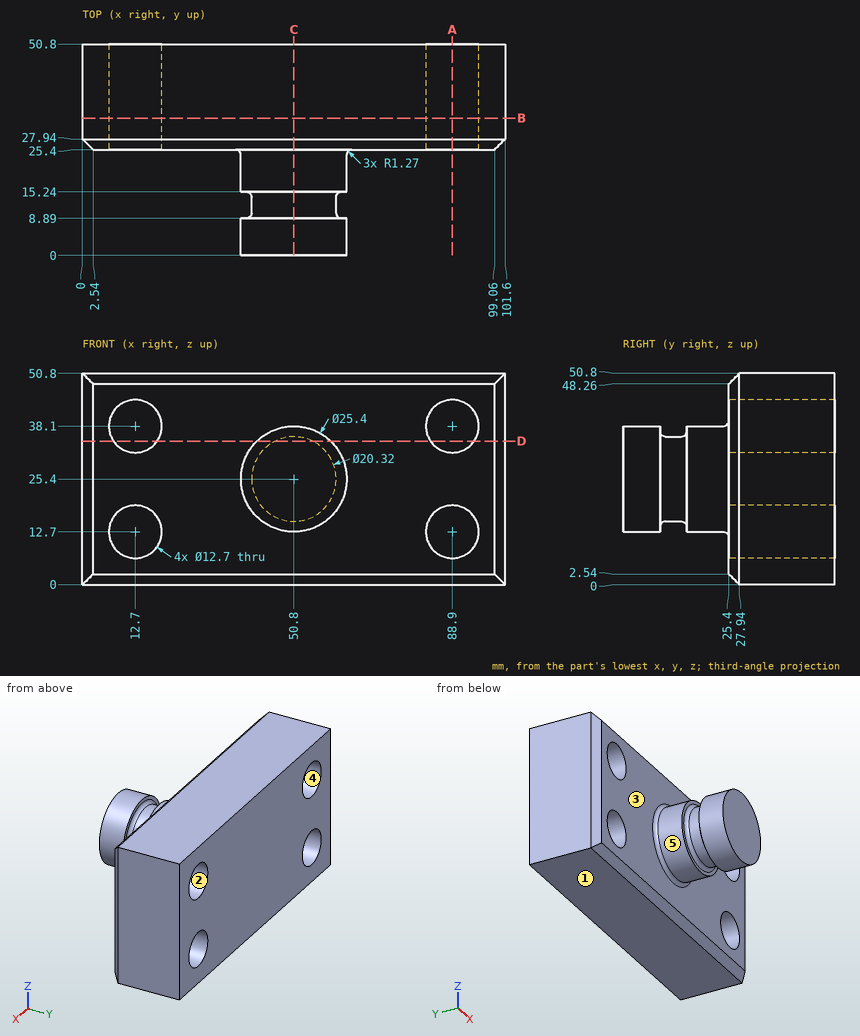
The figure shows three views and two pictorial views of one solid part (mm, origin at its lowest corner). Answer the questions. A direction names the side the tool comes from. Round coordinates to 2 decimals unless told otherwise and drop trailing zeros. Order: outer loops, then holes, each group sorted by start corner. A loop starts at its lowest first (then second) coordinate and runs counter-clockwise, first axis right, second up. Notation, with made-up numbers: (-29.75, 22.25) -> (0.25, 22.25) arc R16 cw to (0.25, 50.25) -> close; hole circle Ø2 at (-31.75, -2). An arc over 180 degrees is marked (long way). Put each result on its own line as item: value.
Q1. Section C-C, the plane x = 50.8 is taken. Write down the section's boundary in (y, z).
Results list:
outline: (0, 12.7) -> (8.89, 12.7) -> (8.89, 13.97) arc R1.27 cw to (10.16, 15.24) -> (13.97, 15.24) arc R1.27 cw to (15.24, 13.97) -> (15.24, 12.7) -> (24.13, 12.7) arc R1.27 cw to (25.4, 11.43) -> (25.4, 2.54) -> (27.94, 0) -> (50.8, 0) -> (50.8, 50.8) -> (27.94, 50.8) -> (25.4, 48.26) -> (25.4, 39.37) arc R1.27 cw to (24.13, 38.1) -> (15.24, 38.1) -> (15.24, 36.83) arc R1.27 cw to (13.97, 35.56) -> (10.16, 35.56) arc R1.27 cw to (8.89, 36.83) -> (8.89, 38.1) -> (0, 38.1) -> close
Q2. Section D-D, the plane z = 34.5 is taken. Count the separate pieces of the cut face and the enclosed holes in it, and give its area (3 significant figures).
Results list:
separate pieces: 3
enclosed holes: 0
area: 2,440 mm^2
Q3. Determine the mould class of the marked faces 1, 2 and 3 for opening direction Z: pulls with the +Z half, pulls with the -Z half, needs draft (parallel to the pull), parting line crosses it, or undercut.
Results list:
face 1: pulls with the -Z half
face 2: undercut
face 3: needs draft
Q4. Which of the six approach directions +Z, -Z, +X, -X, +Y, -Y give full straight-line access (tool end or side, diameter ignored) to the marked faces 4 and 5?
Results list:
face 4: +Y, -Y
face 5: -Y
Q5. This flat-tipped pin is pushed along its axis until it touches: P1, Ø16.5, axis at x = 12.7, z = 38.1, coming from the -Y side. Where does it stop, or does it pass through?
Results list:
P1: y = 25.4
Q6. Section A-A, the plane x = 88.9 is taken. Write down the section's boundary in (y, z), and give its area (3 significant figures).
Results list:
outline: (25.4, 2.54) -> (27.94, 0) -> (50.8, 0) -> (50.8, 6.35) -> (25.4, 6.35) -> close; (25.4, 19.05) -> (50.8, 19.05) -> (50.8, 31.75) -> (25.4, 31.75) -> close; (25.4, 44.45) -> (50.8, 44.45) -> (50.8, 50.8) -> (27.94, 50.8) -> (25.4, 48.26) -> close
area: 639 mm^2
Q7. Consider line 1 along Z through (x, y) = (12.7, 43.75); line 2 along X through (y, z) = (34, 12); line 3 along Z through (x, y) = (93, 47.5). Determine where each line is inside the solid, lowest interval first.
Results list:
line 1: 0 to 6.35, 19.05 to 31.75, 44.45 to 50.8
line 2: 0 to 6.39, 19.01 to 82.59, 95.21 to 101.6
line 3: 0 to 7.85, 17.55 to 33.25, 42.95 to 50.8
Q8. Section B-B, the plane y = 33 is taken. Write down the section's boundary in (x, z).
Results list:
outline: (0, 0) -> (101.6, 0) -> (101.6, 50.8) -> (0, 50.8) -> close; hole circle Ø12.7 at (12.7, 12.7); hole circle Ø12.7 at (12.7, 38.1); hole circle Ø12.7 at (88.9, 12.7); hole circle Ø12.7 at (88.9, 38.1)
